Autodesk Inventor part; units mm, degrees
ref_plane "YZ Plane" through (0, 0, 0) normal (1, 0, 0) x (0, 1, 0)
ref_plane "XZ Plane" through (0, 0, 0) normal (0, 1, 0) x (-1, 0, 0)
ref_plane "XY Plane" through (0, 0, 0) normal (0, 0, 1) x (1, 0, 0)
sketch "Sketch1" plane through (0, 0, 0) normal (0, 1, 0) x (-1, 0, 0)
  line L0 (75, 75) -> (-75, 75)
  line L1 (-75, 75) -> (-75, -75)
  line L2 (-75, -75) -> (75, -75)
  line L3 (75, -75) -> (75, 75)
  circle A0 centre (0, 0) radius 35
  circle A1 centre (65, 65) radius 2.75
  circle A2 centre (-65, 65) radius 2.75
  circle A3 centre (-65, -65) radius 2.75
  circle A4 centre (65, -65) radius 2.75
  point P0 (75, 0)
  point P1 (0, -75)
  dimension "d0" = 150
  dimension "d1" = 150
  dimension "d2" = 70
  dimension "d3" = 5.5
  dimension "d4" = 10
  dimension "d5" = 10
  dimension "d8" = 360
extrude "Extrusion1" add sketch "Sketch1" along normal blind 5
sketch "Sketch2" plane through (0, 0, 0) normal (0, -1, 0) x (1, 0, 0)
  circle A0 centre (0, 0) radius 65
  dimension "d12" = 130
extrude "Extrusion2" cut sketch "Sketch2" against normal blind 10
sketch "Sketch3" plane through (0, 0, 0) normal (0, -1, 0) x (1, 0, 0)
  circle A0 centre (0, 0) radius 65
  circle A1 centre (0, 0) radius 60
  dimension "d15" = 130
  dimension "d16" = 120
extrude "Extrusion3" add sketch "Sketch3" against normal blind 20
sketch "Sketch4" plane through (0, 20, 0) normal (0, 1, 0) x (1, 0, 0)
  circle A0 centre (0, 0) radius 60
  point P0 (0, 0)
  dimension "d42" = 120
extrude "Extrusion4" add sketch "Sketch4" against normal blind 5
sketch "Sketch5" plane through (0, 15, 0) normal (0, -1, 0) x (1, 0, 0)
  circle A0 centre (0, 54) radius 3
  point P0 (0, 0)
  dimension "d21" = 6
  dimension "d22" = 54
extrude "Extrusion5" cut sketch "Sketch5" against normal through all
pattern_circular "Circular Pattern1" count 8 over 360 about axis through (0, 0, 0) along (0, 1, 0) of "Extrusion5"
sketch "Sketch6" plane through (0, 15, 0) normal (0, -1, 0) x (1, 0, 0)
  circle A0 centre (0, 0) radius 7.5
  point P0 (0, 0)
  dimension "d28" = 15
extrude "Extrusion6" cut sketch "Sketch6" against normal blind 10
sketch "Sketch7" plane through (0, 15, 0) normal (0, -1, 0) x (1, 0, 0)
  circle A0 centre (0, 0) radius 45
  circle A1 centre (0, 0) radius 60
  line L0 (0, 0) -> (-26.7546, 36.1827) construction
  circle A2 centre (-38.1838, 38.1838) radius 3
  line L1 (0, 0) -> (-20.4478, 40.086) construction
  circle A3 centre (0, 0) radius 59
  line L2 (-20.4478, 40.086) -> (-26.8093, 52.5572)
  line L3 (-26.7546, 36.1827) -> (-35.0783, 47.4396)
  point P0 (-38.3158, 46.1725)
  point P1 (-27.2637, 53.448)
  dimension "d31" = 15
  dimension "d43" = 120
  dimension "d44" = 118
  dimension "d45" = 14
  dimension "d66" = 8
  dimension "d67" = 170.546
extrude "Extrusion7" add sketch "Sketch7" along normal blind 15 contours A0 L3 A3 L2 picked at (-30.7402, 44.7782)
sketch "Sketch9" plane through (0, 0, 0) normal (0, -1, 0) x (1, 0, 0)
  circle A0 centre (0, 0) radius 29.9834
  circle A1 centre (0, 0) radius 39.9778
  line L0 (0, 0) -> (-26.8767, 13.2908) construction
  line L1 (-35.8356, 17.721) -> (-26.8767, 13.2908)
  point P0 (0, 0)
sketch "Sketch10" plane through (-26.7546, 0, 36.1827) normal (-0.8041, 0, -0.5945) x (-0.5945, 0, 0.8041)
  line L0 (0, 0) -> (14, 0)
  line L1 (14, 0) -> (14, 7.5)
  line L2 (14, 15) -> (14, 0)
  line L3 (0, 15) -> (0, 0)
  line L4 (0, 7.5) -> (14, 7.5)
  line L5 (0, 15) -> (14, 15)
  line L6 (-45, -4) -> (-45, 24)
  point P0 (-45, 0)
  dimension "d46" = 7.5
revolve "Revolution2" add sketch "Sketch10" angle 14 about axis through (0, 0, 0) along (0, -1, 0) contours L3 L4 L1 L0
sketch "Sketch11" plane through (0, 0, 0) normal (0, -1, 0) x (1, 0, 0)
  line L0 (-34.7133, 28.6354) -> (-45.513, 37.5442)
  arc A0 (-20.4478, 40.086) -> (-20.4478, 40.086) centre (0, 0) ccw
  line L1 (-40.1131, 33.0898) -> (-34.7133, 28.6354)
  line L2 (-30.497, 33.0898) -> (-40.1131, 33.0898)
  line L3 (-30.497, 33.0898) -> (-34.7133, 28.6354)
  point P0 (0, 0)
pattern_circular "Circular Pattern2" count 8 over 360 about axis through (0, 0, 0) along (0, 1, 0) of "Extrusion7", "Revolution2"
sketch "Sketch12" plane through (0, 0, 0) normal (0, -1, 0) x (0.7798, 0, 0.626)
  line L0 (-50.9146, -10.5691) -> (-44.0607, -9.1463)
  line L1 (-44.0607, -9.1463) -> (-57.7685, -11.9919)
  arc A0 (-44.8909, -3.1319) -> (-44.0607, -9.1463) centre (0, 0) ccw
  arc A1 (-44.0607, 9.1463) -> (-44.0607, 9.1463) centre (0, 0) ccw
  line L2 (-50.9146, -10.5691) -> (-44.8909, -3.1319)
  line L3 (-50.9146, -10.5691) -> (-44.8909, -3.1319)
  point P0 (0, 0)
extrude "Extrusion9" add sketch "Sketch12" against normal up to surface (7.5 mm away) contours L2 A0 L0
sketch "Sketch13" plane through (0, 20, 0) normal (0, 1, 0) x (1, 0, 0)
  circle A0 centre (0, 0) radius 65
  circle A1 centre (0, 0) radius 61
  dimension "d52" = 4
  dimension "d53" = 130
extrude "Extrusion10" add sketch "Sketch13" along normal blind 13
sketch "Sketch17" plane through (0, 0, 0) normal (0, 0, 1) x (1, 0, 0)
  line L0 (61, 20) -> (-61, 20)
  line L1 (61.0173, 20) -> (-61, 20)
  line L2 (-61, 20) -> (-61, 51.3289)
  line L3 (-61, 51.3289) -> (61.0173, 51.3289)
  line L4 (61.0173, 51.3289) -> (61.0173, 20)
  point P0 (0, 0)
extrude "Extrusion13" cut sketch "Sketch17" along normal through all both and the other way through all
sketch "Sketch14" plane through (0, 33, 0) normal (0, 1, 0) x (1, 0, 0)
  circle A0 centre (0, 0) radius 65
extrude "Extrusion11" add sketch "Sketch14" along normal blind 5
sketch "Sketch18" plane through (0, 20, 0) normal (0, 1, 0) x (1, 0, 0)
  point P0 (0, 0)
sketch "Sketch19" plane through (0, 33, 0) normal (0, -1, 0) x (1, 0, 0)
  circle A0 centre (0, 0) radius 6
  dimension "d63" = 12
extrude "Extrusion14" add sketch "Sketch19" along normal blind 2
sketch "Sketch20" plane through (0, 15, 0) normal (0, -1, 0) x (1, 0, 0)
  circle A0 centre (-38.1838, 38.1838) radius 3
  circle A1 centre (-38.1838, 38.1838) radius 3
  point P0 (0, 0)
  dimension "d68" = 6
extrude "Extrusion15" cut sketch "Sketch20" against normal through all
pattern_circular "Circular Pattern3" count 8 over 360 about axis through (0, 0, 0) along (0, 1, 0) of "Extrusion15"
extrude "Extrusion16" cut sketch "Sketch11" against normal blind 10 contours L0 L2 A0 | A0 L3 picked at (-32.8621, 30.6363)
sketch "Sketch21" plane through (0, 0, 0) normal (0, 0, 1) x (1, 0, 0)
  line L0 (79.7641, 55.8787) -> (-85.0233, 55.8787)
  line L1 (-85.0233, 55.8787) -> (-85.0233, 20)
  line L2 (-85.0233, 20) -> (79.7641, 20)
  line L3 (79.7641, 20) -> (79.7641, 55.8787)
  point P0 (0, 0)
extrude "Extrusion17" cut sketch "Sketch21" along normal through all both and the other way through all
sketch "Sketch23" plane through (0, 15, 0) normal (0, -1, 0) x (1, 0, 0)
  circle A0 centre (-52.6667, -11.9257) radius 1.5
  circle A1 centre (11.9257, -52.6667) radius 1.5
  circle A2 centre (52.6667, 11.9257) radius 1.5
  circle A3 centre (-11.9257, 52.6667) radius 1.5
  circle A4 centre (54, 0) radius 3
  point P0 (0, 0)
  dimension "d79" = 3
  dimension "d82" = 360
  dimension "d93" = 12
  dimension "d94" = 54
extrude "Extrusion18" cut sketch "Sketch23" against normal through all contours A0 | A1 | A2 | A3
sketch "Sketch24" plane through (0, 15, 0) normal (0, -1, 0) x (1, 0, 0)
  circle A0 centre (52.6667, 11.9257) radius 2.5
  circle A1 centre (52.6667, 11.9257) radius 1.5
  circle A2 centre (-11.9257, 52.6667) radius 2.5
  circle A3 centre (-52.6667, -11.9257) radius 2.5
  circle A4 centre (11.9257, -52.6667) radius 2.5
  point P0 (0, 0)
  dimension "d86" = 5
  dimension "d89" = 360
extrude "Extrusion19" cut sketch "Sketch24" against normal blind 2
properties part number "bayonet container 8"
The model under review builds one solid part; all positions refer to its coordinate system, in mm. A direction names the side the tool comes from. Round coordinates to 2 decimals unless told otherwise and drop trailing zeros. Loops run counter-clockwise (first coordinate to the right, second up) from the corner with the lowest first, then second, coordinate; pieces in that order, holes last. Notation, with made-up numbers: (-39, 46) - (0, 46) arc R23 ccw to (0, 66) - close; hole circle Ø5 at (-0.75, 43). An arc over 180 degrees is marked (long way). Use CSV: the item, a comma, the result in double quotes.
(1) Clearance check with flat-ended pins moving along their axes: P1, Ø1.5, axis at x = -53.5, z = -12.5, coming from the -Y side; P2, Ø5.5, axis at x = 12, z = -53, coming from the -Y side; P3, Ø4, axis at y = 12, z = -60, coming from the +X side. State where each tip first meets the part, or that it passes through.
Working result:
P1,"stops at y = 17"
P2,"stops at y = 15"
P3,"stops at x = 29.34"
(2) The part is to be moulded in two halves that separate along Y. For faces 1 (the flat face through (34, 0, 51)), 2 (the flat face through (41.732, 10.938, 30.858)), 3 (the flat face through (-51.665, 3.802, -4.956)), say which applies: pulls with the +Y half, pulls with the -Y half, needs draft (parallel to the pull), parting line crosses it, or undercut.
Working result:
face 1,"pulls with the -Y half"
face 2,"undercut"
face 3,"needs draft"
(3) For line 1 (Z direction, x = 0, y = 6.25); line 2 (Z direction, x = 0, y = 17.65); line 3 (X direction, y = 1, z = 3), list the stretches that pass through material, from the lowest coordinate up.
Working result:
line 1,"z = -65 to -60, -59 to -45, 45 to 59, 60 to 65"
line 2,"z = -65 to -57, -51 to -7.5, 7.5 to 51, 57 to 65"
line 3,"x = -75 to -59.92, -58.92 to -44.9, 44.9 to 58.92, 59.92 to 75"
(4) Take a section at B-B, the plane z = -22.5. Give the boundary of the cut face in (x, y).
Working result:
outline,"(-75, 0) - (-55.62, 0) - (-55.62, 15) - (-44.11, 15) - (-44.11, 0) - (-38.97, 0) - (-38.97, 15) - (55.62, 15) - (55.62, 0) - (75, 0) - (75, 5) - (60.98, 5) - (60.98, 20) - (-60.98, 20) - (-60.98, 5) - (-75, 5) - close"
(5) Take a section at A-A, the plane z = 0. State how many separate pieces and enclosed holes the cut face has, plus the area to 3 significant figures.
Working result:
separate pieces,"6"
enclosed holes,"0"
area,"975 mm^2"
(6) Machinability: for faces 4 (the flat face through (-41.732, 10.938, -30.858)), 5 (the flat face through (-35, 4, 33.09)), 6 (the cylindrical face through (62, 12.4, 19.52)), which of the approach directions +Z, -Z, +X, -X, +Y, -Y give a long, thin tool a straight path to every point of the face, cutting with its end or side? Answer none if there is none.
Working result:
face 4,"none"
face 5,"-Y"
face 6,"+Y"
